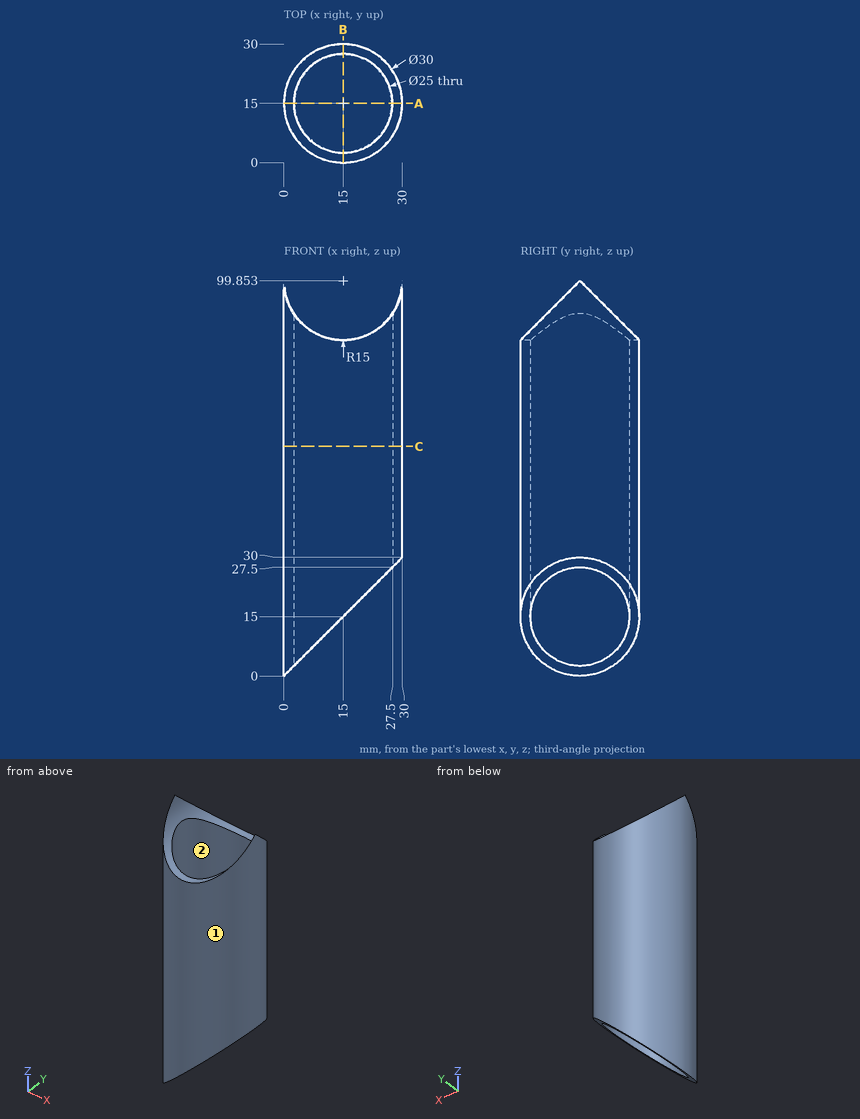
Here's the drawing with two shaded views (mm, measured from the low corner). I have some questions. Coordinates: 2 decimals unless noted, no trailing zeros. Loops run counter-clockwise (first coordinate to the right, second up) from the corner with the lowest first, then second, coordinate; pieces in that order, holes last. Notation, with made-up numbers: (51.25, 12.25) -> (65.25, 12.25) arc R33 ccw to (65.25, 48.25) -> close; hole circle Ø6 at (87.5, 12). An arc over 180 degrees is marked (long way). Answer in a Markdown table with one row per item.
(1) Thinking about a two-plate mould opening in Y: for the marked faces 1 and 2, which applies, released by +Y, released by -Y, zero draft, split by the parting line, or undercut?
Results found:
| item | result |
|---|---|
| face 1 | split by the parting line |
| face 2 | undercut |
(2) Will these pins go through, and if not, where does the flat tip stop? pin 1 Ø3 at (x, y) = (8, 6) entering from +Z; pin 2 Ø10 at (x, y) = (26, 6) entering from +Z; pin 3 Ø1.5 at (x, z) = (18, 56) entering from +Y.
Results found:
| item | result |
|---|---|
| pin 1 | stops at z = 87.49 |
| pin 2 | stops at z = 94.77 |
| pin 3 | stops at y = 29.83 |
(3) If I drill on probe 1 along Y at (x, z) = (15, 72); probe 2 along Y at (x, z) = (21, 29); probe 3 along X at (y, z) = (6, 63.5) (1 decimal), over which ranges is the centre line in solid material (lowest first)?
Results found:
| item | result |
|---|---|
| probe 1 | y = 0 to 2.5, 27.5 to 30 |
| probe 2 | y = 1.25 to 4.03, 25.97 to 28.75 |
| probe 3 | x = 3 to 6.3, 23.7 to 27 |
(4) Imagine slicing it at B-B (x = 15). List the corners of the cut face in (y, z) for me, plus the area to 3 significant figures.
Results found:
| item | result |
|---|---|
| outline | (0, 15) -> (2.5, 15) -> (2.5, 84.85) -> (0, 84.85) -> close; (27.5, 15) -> (30, 15) -> (30, 84.85) -> (27.5, 84.85) -> close |
| area | 349 mm^2 |
(5) Imagine slicing it at A-A (y = 15). List the corners of the cut face in (x, z) for me, plus the area to 3 significant figures.
Results found:
| item | result |
|---|---|
| outline | (0, 0) -> (2.5, 2.5) -> (2.5, 91.56) arc R15 cw to (0, 99.85) -> close; (27.5, 27.5) -> (30, 30) -> (30, 99.85) arc R15 cw to (27.5, 91.56) -> close |
| area | 396 mm^2 |
(6) Imagine slicing it at C-C (z = 58). List the corners of the cut face in (x, y) for me.
Results found:
| item | result |
|---|---|
| outline | circle Ø30 at (15, 15); hole circle Ø25 at (15, 15) |
